Can you work these out from the model? Positions are in its coordinate system, mm. A direction names the side the tool comes from. Round coordinates to 2 decimals unless told otherwise and drop trailing zeros. Loops run counter-clockwise (first coordinate to the right, second up) from the corner with the lowest first, then second, coordinate; pieces in that order, holes last.
(1) Will these pins go through, and if not, where does the flat tip stop? pin 1 Ø15 at (x, y) = (-35, -21) entering from -Z; pin 2 Ø10 at (x, y) = (-44, -5.5) entering from +Z; pin 3 Ø4 at (x, z) = (-46, 4.5) entering from -Y.
(2) I want a section at D-D on x = -32. Write out the boundary of the cut face in (y, z), plus the area to 3 significant figures.
(3) I want a section at A-A on x = -39. Write out the boundary of the cut face in (y, z).
(4) Which directions (+Z, -Z, +X, -X, +Y, -Y) give clear straight access to the entire face, cutting with the end or side of a thin tool? Please do faces 5 (the face through (-45, -4, 2)), 6 (the face through (-37, 1, 2)), 7 (the face through (-49.5, -47.94, -2.46)), 8 (the face through (-49.5, -47.94, 6.54)).
(5) Thinking about a two-plate mould opening in Y: for faces 1 (the face through (-50.112, -45.163, 5.209)), 2 (the face through (-26, -5, 2)), 3 (the face through (-20, -18, 0)), 4 (the face through (-28.55, -24.38, 1.97)), which applies, released by +Y, released by -Y, zero draft, split by the parting line, or undercut?
(6) If I drill on line 1 along Z through (x, y) = (-42.5, -38.5); line 2 along Y through (x, z) = (-36, 3.75); line 3 along X through (y, z) = (-29, 2.75), over which ranges is the centre line in solid material (lowest first)?
from build123d import *

# Parameters (mm, degrees)
F0_W           = 5
F0_H           = 5
F1_DEPTH       = 4
F2_R           = 3
F3_W           = 8
F3_H           = 4
F4_DEPTH       = 2.8
F5_SIZE        = 5
F7_W           = 5.774
F7_H           = 5
F8_DEPTH       = 3
F10_DEPTH      = 25
F10_DEPTH_BACK = 25
F11_DEPTH      = 9
F11_DEPTH_BACK = 5


with BuildPart() as f1:
    # F0 (on Top) → F1 (new body)
    with BuildSketch(Plane.XY):
        Polygon((0, 0), (-40, 0), (-40, -5), (-7.4009361646, -5), (0, -5), align=None)
        Polygon((-51.6094135767, -52.2913145331), (0, -5), (-7.4009361646, -5), (-52.8590282704, -46.6546669079), align=None)
        with Locations((-42.5, -2.5)):
            Rectangle(F0_W, F0_H)
    extrude(amount=F1_DEPTH)

    # F2
    f2_edges = [f1.edges().sort_by_distance(p)[0] for p in [
        (0, 0, 2),
        (0, -5, 2),
    ]]
    fillet(f2_edges, radius=F2_R)

    # F3 (on Front) → F4 (join)
    with BuildSketch(Plane.XZ):
        with Locations((-41, 2)):
            Rectangle(F3_W, F3_H)
    extrude(amount=-F4_DEPTH)

    # F5
    f5_edges = [f1.edges().sort_by_distance(p)[0] for p in [
        (-45, 2.8, 2),
    ]]
    chamfer(f5_edges, length=F5_SIZE)

    # F7 (on offset) → F8 (join)
    with BuildSketch(Plane(origin=(-60.2413457189, -13.3551848163, 0), x_dir=(0.2164396139, -0.9762960071, 0), z_dir=(-0.9762960071, -0.2164396139, 0))):
        with Locations((36.9775523019, 6.5)):
            Rectangle(F7_W, F7_H)
        with Locations((36.9775523019, -2.5)):
            Rectangle(F7_W, F7_H)
    extrude(amount=-F8_DEPTH)

    # F9 (on Top) → F10 (cut, two sides)
    with BuildSketch(Plane.XY) as f10_sk:
        Polygon((-48.0777584016, -51.715362817), (-48.6127237734, -49.5453542475), (-51.6094135767, -52.2913145331), align=None)
    extrude(amount=F10_DEPTH, mode=Mode.SUBTRACT)
    extrude(f10_sk.sketch, amount=-F10_DEPTH_BACK, mode=Mode.SUBTRACT)

    # F9 (on Top) → F11 (join, two sides)
    with BuildSketch(Plane.XY) as f11_sk:
        Polygon((-49.9261649251, -45.9886011426), (-50.3040521353, -44.313404132), (-52.8526316454, -46.6487469866), align=None)
    extrude(amount=F11_DEPTH)
    extrude(f11_sk.sketch, amount=-F11_DEPTH_BACK)


solid = f1.part
Filled sheet:
1. pin 1: stops at z = 0
1. pin 2: stops at z = 4
1. pin 3: stops at y = -48.93
2. outline: (-34.32, 0) - (-27.54, 0) - (-27.54, 4) - (-34.32, 4) - close; (-5, 0) - (0, 0) - (0, 4) - (-5, 4) - close
2. area: 47.1 mm2
3. outline: (-40.74, 0) - (-33.96, 0) - (-33.96, 4) - (-40.74, 4) - close; (-5, 0) - (2.8, 0) - (2.8, 4) - (-5, 4) - close
4. face 5: +Z, -Z, -X, +Y
4. face 6: +Z, -Z, +X, +Y
4. face 7: -Z, +X, +Y
4. face 8: +Z, +X, +Y
5. face 1: released by +Y
5. face 2: undercut
5. face 3: zero draft
5. face 4: undercut
6. line 1: z = 0 to 4
6. line 2: y = -37.99 to -31.21, -5 to 0
6. line 3: x = -33.59 to -26.19
